The listing builds one solid part. Answer for the finished solid, in the listing's coordinates (mm). A direction names the side the tool comes from. Coordinates: 2 decimals unless noted, no trailing zeros. Loops run counter-clockwise (first coordinate to the right, second up) from the corner with the lowest first, then second, coordinate; pieces in that order, holes last. Notation, with made-up numbers: M 32.25,73 L 72.25,73 A24 ccw 72.25,92 Z; hole C -1.5,63 d4. An arc over 180 degrees is marked long. Return JSON: item names as keys, results as strings. Group by question number.
1. Given P1, Ø1, axis at x = 50, z = -16, coming from the +Y side; P2, Ø5, axis at x = 19, z = -7.5, coming from the -Y side; P3, Ø6.5, axis at x = 33.5, y = 0, coming from the -Z side (3 decimals); P4, Ø4, axis at x = 13, z = -19.5, coming from the -Y side (3 decimals), each flat-ended and moving along its own axis, determine where each tip first touches the part or whether it passes through.
2. Section B-B (x = 18) is taken. Write down the section's boundary in (y, z), then the cut area to 3 significant figures.
3. Section A-A (y = 7) is taken. Write down the section's boundary in (x, z), then the cut area to 3 significant figures.
4. The mould has two halves that part along X. Classify faces 5 (the face through (10.65, -8.01, -22.47)), 6 (the face through (53, -8.255, -23)), 7 (the face through (25.4, -6, -21)): pulls with the +X half, pulls with the -X half, needs draft (parallel to the pull), parting line crosses it, or undercut.
5. Straight lines are drawn through the part: L1, parallel to X at y = 6.5, z = -23.75; L2, parallel to X at y = -0.5, z = -4.75; L3, parallel to X at y = 1, z = -22.75. For each, find the intervals that lie inside material, in ascending order. Write a range as from..to.
6. Which of the six approach directions +Z, -Z, +X, -X, +Y, -Y give full straight-line access (tool end or side, diameter ignored) to faces 1 (the face through (51.689, 7, -19)), 2 (the face through (33.147, 0, -18)), 3 (the face through (37, 0, -9.779)), 4 (the face through (55, -1.397, -21))?
```python
from build123d import *

# Parameters (mm, degrees)
BOSS_EXTRUDE1_DEPTH    = 34.29
SKETCH2_W              = 4.699
SKETCH2_H              = 1.424459459
SKETCH2_H_2            = 0.480540541
CUT_EXTRUDE1_DEPTH     = 60.774381845
SKETCH3_W              = 3.175
SKETCH3_H              = 4.572
CUT_EXTRUDE2_DEPTH     = 9.779
CUT_EXTRUDE3_DEPTH     = 70.085665402
CUT_EXTRUDE4_START     = -17.78
CUT_EXTRUDE4_OUTLINE_W = 7.62
CUT_EXTRUDE4_OUTLINE_H = 4.7625
CUT_EXTRUDE4_DEPTH     = 17.78
SKETCH6_W              = 10.915170011
SKETCH6_H              = 18.687954265
CUT_EXTRUDE5_DEPTH     = 74.422
CUT_EXTRUDE6_DEPTH     = 74.422
FILLET2_R              = 0.508
FILLET3_R              = 2.54


# Read off the part's stored shape, not the designer's step: Cut-Extrude4
with BuildPart() as part:
    # Sketch1 → Boss-Extrude1 (new body)
    with BuildSketch(Plane.XY):
        Polygon((9.398, 6.35), (9.398, -6.35), (9.398, -7.774459459), (11.938, -8.255), (11.938, -6.35), (51.689, -6.35), (51.689, -8.255), (54.483, -8.255), (54.483, -3.4925), (57.658, -3.4925), (57.658, 3.4925), (54.483, 3.4925), (54.483, 8.255), (51.689, 8.255), (51.689, 6.35), (11.938, 6.35), (11.938, 8.255), (9.398, 7.774459459), align=None)
    extrude(amount=-BOSS_EXTRUDE1_DEPTH)

    # Sketch2 → Cut-Extrude1 (cut, through all)
    with BuildSketch(Plane.ZY.offset(-9.398)):
        with BuildLine():
            ThreePointArc((11.962240433, -0.310327796), (7.428822396, 6.001266395), (0, 3.720762472))
            Line((0, 3.720762472), (0, 0.889))
            ThreePointArc((0, 0.889), (6.395096144, 1.80805092), (11.813233179, -1.711281452))
            ThreePointArc((11.813233179, -1.711281452), (11.924883856, -1.014755633), (11.962240433, -0.310327796))
        make_face()
        with BuildLine():
            Line((0, 0.889), (0, 3.720762472))
            ThreePointArc((0, 3.720762472), (-0.961463724, 1.954640839), (-1.351994264, -0.017942243))
            ThreePointArc((-1.351994264, -0.017942243), (-0.696131125, 0.465542965), (0, 0.889))
        make_face()
        with BuildLine():
            ThreePointArc((0, 0.889), (-0.696131125, 0.465542965), (-1.351994264, -0.017942243))
            ThreePointArc((-1.351994264, -0.017942243), (-1.054856668, -2.298153331), (0, -4.341418064))
            Line((0, -4.341418064), (0, 0.889))
        make_face()
        with BuildLine():
            ThreePointArc((11.813233179, -1.711281452), (6.395096144, 1.80805092), (0, 0.889))
            Line((0, 0.889), (0, -4.341418064))
            ThreePointArc((0, -4.341418064), (6.749348825, -6.811473452), (11.813233179, -1.711281452))
        make_face()
        with BuildLine():
            ThreePointArc((0, -4.341418064), (-1.054856668, -2.298153331), (-1.351994264, -0.017942243))
            ThreePointArc((-1.351994264, -0.017942243), (-3.994827922, -3.482124307), (-4.743817945, -7.774459459))
            Line((-4.743817945, -7.774459459), (0, -7.774459459))
            Line((0, -7.774459459), (0, -4.341418064))
        make_face()
        with Locations((-2.3495, 7.06222973)):
            Rectangle(SKETCH2_W, SKETCH2_H)
        with Locations((-2.3495, 8.01472973)):
            Rectangle(SKETCH2_W, SKETCH2_H_2)
        with BuildLine():
            Line((0, -7.774459459), (-4.743817945, -7.774459459))
            ThreePointArc((-4.743817945, -7.774459459), (-4.72456581, -8.015024154), (-4.699, -8.255))
            Line((-4.699, -8.255), (0, -8.255))
            Line((0, -8.255), (0, -7.774459459))
        make_face()
    extrude(amount=-CUT_EXTRUDE1_DEPTH, mode=Mode.SUBTRACT)

    # Sketch3 → Cut-Extrude2 (cut)
    with BuildSketch(Plane.XY):
        with Locations((36.7665, -0.381)):
            Rectangle(SKETCH3_W, SKETCH3_H)
    extrude(amount=-CUT_EXTRUDE2_DEPTH, mode=Mode.SUBTRACT)

    # Sketch4 → Cut-Extrude3 (cut, through all)
    with BuildSketch(Plane.XZ.offset(8.255)):
        with BuildLine():
            Line((51.689, -34.29), (51.689, -16.51))
            Line((51.689, -16.51), (40.767, -16.51))
            Line((40.767, -16.51), (40.767, -19.431))
            ThreePointArc((40.767, -19.431), (40.320630735, -20.508630735), (39.243, -20.955))
            Line((39.243, -20.955), (34.671, -20.955))
            ThreePointArc((34.671, -20.955), (33.593369265, -20.508630735), (33.147, -19.431))
            Line((33.147, -19.431), (33.147, -16.51))
            Line((33.147, -16.51), (25.4, -16.51))
            Line((25.4, -16.51), (25.4, -25.4))
            Line((25.4, -25.4), (15.875, -25.4))
            Line((15.875, -25.4), (15.875, -16.51))
            Line((15.875, -16.51), (15.748, -16.51))
            ThreePointArc((15.748, -16.51), (13.053923164, -17.625923164), (11.938, -20.32))
            Line((11.938, -20.32), (11.938, -34.29))
            Line((11.938, -34.29), (51.689, -34.29))
        make_face()
        with BuildLine():
            Line((35.179, -16.51), (38.354, -16.51))
            Line((38.354, -16.51), (38.354, -18.288))
            ThreePointArc((38.354, -18.288), (38.130815367, -18.826815367), (37.592, -19.05))
            Line((37.592, -19.05), (35.941, -19.05))
            ThreePointArc((35.941, -19.05), (35.402184633, -18.826815367), (35.179, -18.288))
            Line((35.179, -18.288), (35.179, -16.51))
        make_face()
        Polygon((57.658, -4.699), (54.483, -4.699), (51.562, 0), (57.658, 0), align=None)
        Polygon((6.604, -4.699), (12.319, -4.699), (24.892, 0), (6.604, 0), align=None)
    extrude(amount=-CUT_EXTRUDE3_DEPTH, mode=Mode.SUBTRACT)

    # Cut-Extrude4 outline → Cut-Extrude4 (cut)
    with BuildSketch(Plane(origin=(0, 0, -34.29), x_dir=(-1, 0, 0), z_dir=(0, 0, -1)).offset(CUT_EXTRUDE4_START)):
        with BuildLine():
            Line((-22.225, -6.35), (-15.875, -6.35))
            Line((-15.875, -6.35), (-15.875, -5.021000706))
            Line((-15.875, -5.021000706), (-11.938, -5.021000706))
            Line((-11.938, -5.021000706), (-9.906, -4.636568273))
            Line((-9.906, -4.636568273), (-9.906, 4.636568273))
            Line((-9.906, 4.636568273), (-11.938, 5.021000706))
            Line((-11.938, 5.021000706), (-15.875, 5.021000706))
            Line((-15.875, 5.021000706), (-15.875, 6.35))
            Line((-15.875, 6.35), (-22.225, 6.35))
            ThreePointArc((-22.225, 6.35), (-15.875, 0), (-22.225, -6.35))
        make_face()
        with Locations((-36.957, -3.96875)):
            Rectangle(CUT_EXTRUDE4_OUTLINE_W, CUT_EXTRUDE4_OUTLINE_H)
        with BuildLine():
            Line((-25.4, 4.7752), (-25.4, -4.7752))
            Line((-25.4, -4.7752), (-22.225, -4.7752))
            ThreePointArc((-22.225, -4.7752), (-17.4498, 0), (-22.225, 4.7752))
            Line((-22.225, 4.7752), (-25.4, 4.7752))
        make_face()
        with Locations((-36.957, 3.96875)):
            Rectangle(CUT_EXTRUDE4_OUTLINE_W, CUT_EXTRUDE4_OUTLINE_H)
        Polygon((-54.181998462, -1.397), (-51.689, -5.715), (-51.689, 5.715), (-54.181998462, 1.397), (-55.753, 1.397), (-55.753, -1.397), align=None)
    extrude(amount=CUT_EXTRUDE4_DEPTH, mode=Mode.SUBTRACT)

    # Sketch6 → Cut-Extrude5 (cut)
    with BuildSketch(Plane.ZY.offset(-9.398)):
        with Locations((-31.703953975, 0.006721575)):
            Rectangle(SKETCH6_W, SKETCH6_H)
    extrude(amount=-CUT_EXTRUDE5_DEPTH, mode=Mode.SUBTRACT)

    # Sketch7 → Cut-Extrude6 (cut)
    with BuildSketch(Plane.ZY.offset(-9.398)):
        Polygon((-19.4945, 8.255), (-19.4945, 8.707804747), (-4.699, 8.83298433), (3.124174595, 8.83298433), (3.124174595, 5.342724301), (3.124174595, 4.343051296), align=None)
        Polygon((3.124174595, -4.343051296), (3.124174595, -5.342724301), (3.124174595, -8.83298433), (-4.699, -8.83298433), (-19.4945, -8.707804747), (-19.4945, -8.255), align=None)
    extrude(amount=-CUT_EXTRUDE6_DEPTH, mode=Mode.SUBTRACT)

    # Fillet2
    fillet2_edges = [part.edges().sort_by_distance(p)[0] for p in [
        (38.227, 4.883384051, 0),
    ]]
    fillet(fillet2_edges, radius=FILLET2_R)

    # Fillet3
    fillet3_edges = [part.edges().sort_by_distance(p)[0] for p in [
        (45.378214433, -0.017942243, -1.351994264),
        (28.226750917, -0.017942243, -1.351994264),
    ]]
    fillet(fillet3_edges, radius=FILLET3_R)


solid = part.part
```
Worked out:
{
 "1": {"P1": "y = 6.35", "P2": "y = -6.35", "P3": "z = -20.955", "P4": "y = -8.255"},
 "2": {"outline": "M -6.35,-16.51 L -4.74,-16.51 L -4.74,-25.4 L -2.23,-25.4 L -2.23,-16.51 L 2.23,-16.51 L 2.23,-25.4 L 4.74,-25.4 L 4.74,-16.51 L 6.35,-16.51 L 6.35,-8.48 L 5.33,-2.58 L -1.21,-2.58 A9.18 cw -5.69,-4.64 L -6.35,-8.48 Z", "area": "210 mm^2"},
 "3": {"outline": "M 9.4,-26.25 L 11.94,-26.25 L 11.94,-12.24 L 9.4,-12.24 Z; M 51.69,-26.25 L 54.48,-26.25 L 54.48,-12.24 L 51.69,-12.24 Z", "area": "74.7 mm^2"},
 "4": {"face 5": "pulls with the -X half", "face 6": "needs draft", "face 7": "undercut"},
 "5": {"L1": "9.4..11.94, 51.69..54.48", "L2": "9.4..35.18, 38.35..57.66", "L3": "9.4..9.91, 15.95..17.56, 55.75..57.66"},
 "6": {"face 1": "-Z, +Y", "face 2": "-Z, +Y, -Y", "face 3": "+Z", "face 4": "-Z"}
}
